Autodesk Inventor part; units mm, degrees
ref_plane "YZ Plane" through (0, 0, 0) normal (1, 0, 0) x (0, 1, 0)
ref_plane "XZ Plane" through (0, 0, 0) normal (0, 1, 0) x (-1, 0, 0)
ref_plane "XY Plane" through (0, 0, 0) normal (0, 0, 1) x (1, 0, 0)
sketch "Sketch1" plane through (0, 0, 0) normal (0, 1, 0) x (-1, 0, 0)
  line L0 (3.175, 0) -> (85.725, 0)
  line L1 (88.9, -3.175) -> (88.9, -34.925)
  line L2 (85.725, -38.1) -> (3.175, -38.1)
  line L3 (0, -34.925) -> (0, -3.175)
  arc A0 (88.9, -3.175) -> (85.725, 0) centre (85.725, -3.175) ccw
  arc A1 (85.725, -38.1) -> (88.9, -34.925) centre (85.725, -34.925) ccw
  arc A2 (0, -34.925) -> (3.175, -38.1) centre (3.175, -34.925) ccw
  arc A3 (3.175, 0) -> (0, -3.175) centre (3.175, -3.175) ccw
  point P0 (0, 0)
  point P1 (88.9, -38.1)
  point P2 (88.9, 0)
  point P3 (0, -38.1)
  dimension "d0" = 88.9
  dimension "d1" = 38.1
  dimension "d2" = 3.175
extrude "Extrusion1" add sketch "Sketch1" along normal blind 914.4
sketch "Sketch2" plane through (-85.725, 0, 0) normal (0, 0, 1) x (1, 0, 0)
  line L0 (0, 0) -> (82.55, 0) construction
  line L1 (82.55, 0) -> (82.55, 914.4) construction
  line L2 (0, 914.4) -> (82.55, 914.4) construction
  line L3 (0, 0) -> (0, 914.4) construction
  line L4 (-3.175, 0) -> (-3.175, 914.4) construction
  line L5 (85.725, 0) -> (85.725, 914.4) construction
  circle A0 centre (41.275, 44.45) radius 7.3025
  line L6 (41.275, 0) -> (41.275, 44.45) construction
  line L7 (41.275, 44.45) -> (-3.175, 44.45) construction
  line L8 (-3.175, 0) -> (-3.175, 914.4) construction
  line L9 (-3.175, 457.2) -> (85.725, 457.2) construction
  circle A1 centre (41.275, 869.95) radius 7.3025
  dimension "d5" = 14.605
extrude "Extrusion2" cut sketch "Sketch2" against normal through all
sketch "Sketch3" plane through (-85.725, 0, -38.1) normal (0, 0, 1) x (1, 0, 0)
  circle A0 centre (41.275, 44.45) radius 7.3025
  circle A1 centre (41.275, 44.45) radius 12.7
  line L0 (0, 0) -> (0, 914.4) construction
  line L1 (0, 457.2) -> (82.55, 457.2) construction
  line L2 (82.55, 0) -> (82.55, 914.4) construction
  circle A2 centre (41.275, 869.95) radius 12.7
  point P0 (85.725, 0)
  dimension "d8" = 25.4
extrude "Extrusion3" cut sketch "Sketch3" along normal blind 12.7 contours A0 | A1 | A2
sketch "Sketch4" plane through (-85.725, 0, 0) normal (0, 0, 1) x (1, 0, 0)
  line L0 (85.725, 0) -> (-3.175, 0) construction
  line L1 (-3.175, 0) -> (-3.175, 38.1) construction
  line L2 (-3.175, 38.1) -> (85.725, 38.1) construction
  line L3 (85.725, 38.1) -> (85.725, 0) construction
  circle A0 centre (66.675, 19.05) radius 19.05 construction
  line L4 (0, 0) -> (82.55, 0)
  circle A1 centre (15.875, 19.05) radius 19.05 construction
  circle A2 centre (66.675, 19.05) radius 1.5875
  circle A3 centre (15.875, 19.05) radius 1.5875
  circle A4 centre (41.275, 19.05) radius 1.5875
  line L5 (0, 0) -> (0, 914.4)
  line L6 (0, 457.2) -> (82.55, 457.2) construction
  line L7 (82.55, 0) -> (82.55, 914.4)
  line L8 (85.725, 438.15) -> (-3.175, 438.15) construction
  line L9 (-3.175, 438.15) -> (-3.175, 476.25) construction
  line L10 (-3.175, 476.25) -> (85.725, 476.25) construction
  line L11 (85.725, 476.25) -> (85.725, 438.15) construction
  circle A5 centre (66.675, 457.2) radius 19.05 construction
  circle A6 centre (15.875, 457.2) radius 19.05 construction
  circle A7 centre (66.675, 457.2) radius 1.5875
  circle A8 centre (15.875, 457.2) radius 1.5875
  circle A9 centre (41.275, 457.2) radius 1.5875
  circle A10 centre (66.675, 895.35) radius 1.5875
  circle A11 centre (15.875, 895.35) radius 1.5875
  circle A12 centre (41.275, 895.35) radius 1.5875
  point P0 (41.275, 0)
  point P1 (41.275, 438.15)
  point P2 (41.275, 457.2)
  dimension "d11" = 88.9
  dimension "d12" = 38.1
  dimension "d13" = 3.175
  dimension "d14" = 88.9
  dimension "d15" = 38.1
  dimension "d16" = 3.175
extrude "Extrusion4" cut sketch "Sketch4" against normal through all
properties part number "Horizontal Beam 3ft" material "Wood (Birch)"
For this review, take the finished solid that the model builds, in its own axes (mm). A direction names the side the tool comes from. Give positions to 0.01 mm unless a question says otherwise; leave off trailing zeros.
1) The part is to be moulded in two halves that separate along X. For faces 3 (the face through (-44, 914.4, -19)), 4 (the face through (-88.9, 451, -19)), 5 (the face through (-39, 864, -25.4)), 6 (the face through (-46.103, 857.358, -31.839)), say which applies: released by +X, released by -X, zero draft, split by the parting line, or undercut.
2) Insertion check: pin 1 (20.5 mm diameter, centred on x = -44.45, y = 869.95, fed in from -Z). The pin has a flat end and moves straight along its axis. Give the tip position at first contact, or say it passes through.
3) For faces 1 (the face through (-39, 39, -25.4)), 2 (the face through (-41.08, 863.47, -12.52)), list the 3-axis set-ups (+Z, -Z, +X, -X, +Y, -Y) from which the entire face can be reached by the end or side of a thin tool; tool diameter is ignored.
4) Wall thickness on line 1 (Y direction, x = -19.05, z = -15.5); line 2 (X direction, y = 457, z = -27); line 3 (Y direction, x = -44, z = -21): over which ranges is each line inside the solid? List them lowest first.
Derived:
1. face 3: zero draft
1. face 4: released by -X
1. face 5: undercut
1. face 6: undercut
2. pin 1: stops at z = -25.4
3. face 1: -Z
3. face 2: +Z, -Z
4. line 1: y = 0 to 17.46, 20.64 to 455.61, 458.79 to 893.76, 896.94 to 914.4
4. line 2: x = -88.9 to -71.42, -68.28 to -46.02, -42.88 to -20.62, -17.48 to 0
4. line 3: y = 0 to 17.53, 20.57 to 37.16, 51.74 to 455.68, 458.72 to 862.66, 877.24 to 893.83, 896.87 to 914.4
